Can you work these out from the model? Positions are in its coordinate system, mm. Face numbers are marked on the shaded views. A direction names the side the tool comes from. Coordinates: 2 decimals unless noted, no trailing zeros. Write each loop counter-clockwise with the first axis right and the second up, starting at its lowest first coordinate (ties: lowest second). Pieces come first, ordered by that corner, then holes. Notation, with made-up numbers: (46, 49.25) - (86, 49.25) arc R26 cw to (86, 74.25) - close; hole circle Ø7 at (-21.5, 12). An arc over 180 degrees is marked (long way). Use one line per item in the form item = value. Start each with the question number.
(1) If we section it at A-A on x = 0: Please give me the cut outline in (y, z), then the cut area to 3 significant figures.
(2) If we section it at B-B on y = 9: Please give me the cut outline in (x, z), then the cut area to 3 significant figures.
(3) If we section it at C-C on y = 4: Please give me the cut outline in (x, z).
(4) If I drill on probe 1 along Y at (x, z) = (0.75, -2); probe 2 along Z at (x, y) = (-2, 9); probe 3 along Z at (x, y) = (-2.5, 9.75), over which ranges is the centre line in solid material (lowest first)? Write a range as from..to.
(5) On a 3-axis mill with a long thin cutter (end or side, diameter ignored), from which of +Z, -Z, +X, -X, +Y, -Y can I reach the whole of each face in a straight line? I mean the marked faces 1 and 2. Say none if no direction works.
(6) For pin 1 Ø1 at (x, y) = (-1, 3) entering from -Z; pin 2 Ø3 at (x, y) = (-2, 3) entering from +Z; pin 3 Ø1.5 at (x, z) = (1, 0.5) entering from +Y, each with a flat end and sliding along its axis, tell me the tip position at first contact or that it passes through.
(7) Thinking about a two-plate mould opening in Z: for the marked faces 3, 4 and 5, which applies, pulls with the +Z half, pulls with the -Z half, needs draft (parallel to the pull), parting line crosses it, or undercut?
(8) If we section it at D-D on y = 2.5: Please give me the cut outline in (x, z).
```python
from build123d import *

# Parameters (mm, degrees)
SKETCH2_R           = 4
BOSS_EXTRUDE1_DEPTH = 10
CUT_EXTRUDE1_DEPTH  = 1.5
CHAMFER1_SIZE       = 0.5
CHAMFER2_SIZE       = 1
CHAMFER2_SIZE2      = 2.747477419


with BuildPart() as part:
    # Sketch2 → Boss-Extrude1 (new body)
    with BuildSketch(Plane(origin=(0, 0, 0), x_dir=(1, 0, 0), z_dir=(0, 1, 0))):
        with Locations(Location((0, 0, 0), (0, 0, 270))):
            Circle(SKETCH2_R)
    extrude(amount=BOSS_EXTRUDE1_DEPTH)

    # Sketch3 → Cut-Extrude1 (cut)
    with BuildSketch(Plane(origin=(0, 10, 0), x_dir=(1, 0, 0), z_dir=(0, 1, 0))):
        Polygon((2.886751346, 0), (1.443375673, 2.5), (-1.443375673, 2.5), (-2.886751346, 0), (-1.443375673, -2.5), (1.443375673, -2.5), align=None)
    extrude(amount=-CUT_EXTRUDE1_DEPTH, mode=Mode.SUBTRACT)

    # Chamfer1
    chamfer1_edges = [part.edges().sort_by_distance(p)[0] for p in [
        (0, 10, -4),
    ]]
    chamfer(chamfer1_edges, length=CHAMFER1_SIZE)

    # Chamfer2
    chamfer2_edges = [part.edges().sort_by_distance(p)[0] for p in [
        (0, 0, -4),
    ]]
    chamfer2_side = [part.faces().sort_by_distance(p)[0] for p in [
        (0, 0, 0),
    ]]
    chamfer(chamfer2_edges, length=CHAMFER2_SIZE, length2=CHAMFER2_SIZE2, reference=chamfer2_side[0])


solid = part.part
```
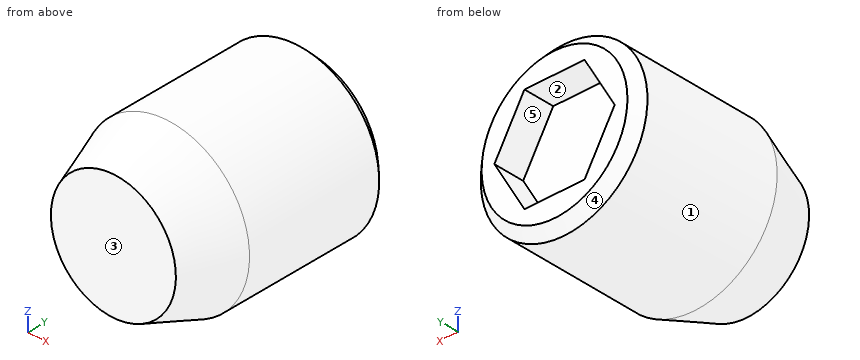
Reported:
q1.outline = (0, -3) - (2.75, -4) - (9.5, -4) - (10, -3.5) - (10, -2.5) - (8.5, -2.5) - (8.5, 2.5) - (10, 2.5) - (10, 3.5) - (9.5, 4) - (2.75, 4) - (0, 3) - close
q1.area = 69.5 mm2
q2.outline = circle Ø8 at (0, 0); hole (-2.89, 0) - (-1.44, -2.5) - (1.44, -2.5) - (2.89, 0) - (1.44, 2.5) - (-1.44, 2.5) - close
q2.area = 28.6 mm2
q3.outline = circle Ø8 at (0, 0)
q4.probe_1 = 0..8.5
q4.probe_2 = -3.46..-1.54, 1.54..3.46
q4.probe_3 = -2.8..-0.67, 0.67..2.8
q5.face_1 = +Y, -Y
q5.face_2 = +Y
q6.pin_1 = -3.97
q6.pin_2 = 3.97
q6.pin_3 = 8.5
q7.face_3 = needs draft
q7.face_4 = parting line crosses it
q7.face_5 = undercut
q8.outline = circle Ø7.82 at (0, 0)
